Here's how the part is built. I have some questions about the finished solid (model axes, mm). A direction names the side the tool comes from. Give positions to 0.01 mm unless a question says otherwise; leave off trailing zeros. Order: outer loops, then holes, each group sorted by start corner. A loop starts at its lowest first (then second) coordinate and runs counter-clockwise, first axis right, second up.
from build123d import *

# Parameters (mm, degrees)
BOSS_EXTRUDE1_DEPTH = 38.1
SHELL1_T            = -3.81
CUT_EXTRUDE1_DEPTH  = 3.81
BOSS_EXTRUDE2_DEPTH = 101.6
SKETCH5_W           = 24.13
SKETCH5_H           = 30.48
CUT_EXTRUDE2_DEPTH  = 97.79
BOSS_EXTRUDE3_DEPTH = 25.4
SKETCH9_W           = 44.45
SKETCH9_H           = 19.05
CUT_EXTRUDE4_DEPTH  = 76.2


with BuildPart() as part:
    # Sketch1 → Boss-Extrude1 (new body)
    with BuildSketch(Plane.XY):
        Polygon((0, 0), (25.4, 0), (25.4, 5.08), (5.08, 101.6), (0, 101.6), align=None)
    extrude(amount=BOSS_EXTRUDE1_DEPTH)

    # Shell1
    shell1_openings = [part.faces().sort_by_distance(p)[0] for p in [
        (15.24, 53.34, 19.05),
    ]]
    offset(amount=SHELL1_T, openings=shell1_openings, kind=Kind.INTERSECTION)

    # Sketch2 → Cut-Extrude1 (cut)
    with BuildSketch(Plane.XZ):
        with BuildLine():
            Line((6.35, 22.225), (19.05, 22.225))
            ThreePointArc((19.05, 22.225), (22.225, 19.05), (19.05, 15.875))
            Line((19.05, 15.875), (6.35, 15.875))
            ThreePointArc((6.35, 15.875), (3.175, 19.05), (6.35, 22.225))
        make_face()
    extrude(amount=-CUT_EXTRUDE1_DEPTH, mode=Mode.SUBTRACT)

    # Sketch3 → Boss-Extrude2 (add)
    with BuildSketch(Plane(origin=(0, 101.6, 0), x_dir=(1, 0, 0), z_dir=(0, 1, 0))):
        Polygon((-19.05, 0), (0, -19.05), (0, 0), align=None)
        Polygon((0, -38.1), (0, -19.05), (-19.05, -38.1), align=None)
    extrude(amount=-BOSS_EXTRUDE2_DEPTH)

    # Sketch5 → Cut-Extrude2 (cut)
    with BuildSketch(Plane(origin=(0, 101.6, 0), x_dir=(1, 0, 0), z_dir=(0, 1, 0))):
        with Locations((13.335, -19.05)):
            Rectangle(SKETCH5_W, SKETCH5_H)
    extrude(amount=-CUT_EXTRUDE2_DEPTH, mode=Mode.SUBTRACT)

    # Sketch6 → Boss-Extrude3 (add)
    with BuildSketch(Plane.XZ):
        Polygon((-19.05, 0), (0, 19.05), (-19.05, 38.1), align=None)
    extrude(amount=-BOSS_EXTRUDE3_DEPTH)

    # Sketch9 → Cut-Extrude4 (cut)
    with BuildSketch(Plane(origin=(0, 101.6, 0), x_dir=(1, 0, 0), z_dir=(0, 1, 0))):
        with Locations((3.175, -9.525)):
            Rectangle(SKETCH9_W, SKETCH9_H)
    extrude(amount=-CUT_EXTRUDE4_DEPTH, mode=Mode.SUBTRACT)


solid = part.part
Q1. If we section it at A-A on x = 10: List the corners of the cut face in (y, z) for me (3 decimals).
Filled sheet:
outline: (0, 0) - (25.4, 0) - (25.4, 3.81) - (3.81, 3.81) - (3.81, 15.875) - (0, 15.875) - close; (0, 22.225) - (3.81, 22.225) - (3.81, 34.29) - (78.23, 34.29) - (78.23, 38.1) - (0, 38.1) - close
Q2. If we section it at D-D on y = 12: List the corners of the cut face in (x, z) for me.
Filled sheet:
outline: (-19.05, 0) - (23.94, 0) - (23.94, 3.81) - (1.27, 3.81) - (1.27, 34.29) - (23.94, 34.29) - (23.94, 38.1) - (-19.05, 38.1) - close
Q3. If we section it at C-C on x = -6: List the corners of the cut face in (y, z) for me.
Filled sheet:
outline: (0, 0) - (25.4, 0) - (25.4, 25.05) - (101.6, 25.05) - (101.6, 38.1) - (0, 38.1) - close
Q4. I'm going to push flat-ended pins straight in: P1, Ø5, axis at x = 11.5, z = 24.5, coming from the -Y side; P2, Ø4, axis at y = 63, z = 29, coming from the +X side; P3, Ø10, axis at x = 17, y = 82, coming from the -Z side (3 decimals); P4, Ø2, axis at x = 14.5, z = 28, coming from the +Y side. Where does each tip first touch, or does it pass through?
Filled sheet:
P1: stops at y = 0
P2: stops at x = 1.27
P3: passes through
P4: stops at y = 3.81
Q5. Thinking about a two-plate mould opening in X: for faces 5 (the face through (13, 2, 22.225)), 6 (the face through (-2, 52, 38.1)), 7 (the face through (23.29, 15.1, 1.88)), 8 (the face through (-9.39, 64.03, 28.44)), which applies, released by +X, released by -X, zero draft, split by the parting line, or undercut?
Filled sheet:
face 5: undercut
face 6: zero draft
face 7: released by +X
face 8: released by -X
Q6. For faces 1 (the face through (3, 0, 19)), 2 (the face through (-8, 25.4, 11)), 3 (the face through (22.224, 1.878, 19.12)), 4 (the face through (10, 43, 34.29)), which set-ups out of +Z, -Z, +X, -X, +Y, -Y let a thin tool reach every point of the face, with its end or its side?
Filled sheet:
face 1: +Z, -Z, +X, -X, -Y
face 2: -Z, -X, +Y
face 3: +Y, -Y
face 4: +X, +Y
Q7. If we section it at B-B on z = 29: List the corners of the cut face in (x, y) for me, plus the area to 3 significant figures.
Filled sheet:
outline: (-19.05, 0) - (25.4, 0) - (25.4, 3.81) - (1.27, 3.81) - (1.27, 101.6) - (-9.95, 101.6) - (-9.95, 25.4) - (-19.05, 25.4) - close
area: 1,460 mm2
Q8. I need wall thicknesses on L1, parallel to Z at x = 14, y = 7.5; L2, parallel to Z at x = 10, y = 63.5; L3, parallel to X at y = 9.5, z = 12.5. Which ranges of each line are inside material? Lowest first, please.
Filled sheet:
L1: z = 0 to 3.81, 34.29 to 38.1
L2: z = 34.29 to 38.1
L3: x = -19.05 to 1.27
